from build123d import *

# Parameters (mm, degrees)
ESBO_O1_R                = 6.85
RESSALTO_EXTRUS_O1_DEPTH = 3.2
ESBO_O3_R                = 5.8
RESSALTO_EXTRUS_O2_DEPTH = 15
ESBO_O3_2_R              = 5.8
RESSALTO_EXTRUS_O3_DEPTH = 15


with BuildPart() as part:
    # Esbo_o1 → Ressalto-extrus_o1 (new body)
    with BuildSketch(Plane(origin=(0, 0, 0), x_dir=(1, 0, 0), z_dir=(0, 1, 0))):
        with Locations(Location((0, 0, 0), (0, 0, 270))):
            Circle(ESBO_O1_R)
    extrude(amount=RESSALTO_EXTRUS_O1_DEPTH)

    # Esbo_o3 → Ressalto-extrus_o2 (add)
    with BuildSketch(Plane.XZ):
        with Locations(Location((0, 0, 0), (0, 0, 270))):
            Circle(ESBO_O3_R)
    extrude(amount=RESSALTO_EXTRUS_O2_DEPTH)

    # Esbo_o3_2 → Ressalto-extrus_o3 (add)
    with BuildSketch(Plane.XZ):
        with Locations(Location((0, 0, 0), (0, 0, 270))):
            Circle(ESBO_O3_2_R)
    extrude(amount=RESSALTO_EXTRUS_O3_DEPTH)


solid = part.part
For this review, take the finished solid that the model builds, in its own axes (mm). A direction names the side the tool comes from. Give positions to 0.01 mm unless a question says otherwise; leave off trailing zeros. Loops run counter-clockwise (first coordinate to the right, second up) from the corner with the lowest first, then second, coordinate; pieces in that order, holes last.
Item 1: Take a section at A-A, the plane x = 0. State the section outline as (y, z) points.
Item 2: For line 1 along Y through (x, z) = (-5.5, 2.25); line 2 along Z through (x, y) = (1, 1.25); line 3 along X through (y, z) = (-0.5, 4.5), list the stretches that pass through material, from the lowest coordinate up.
Item 3: Tool access review of faces 1 (the flat face through (2, 0, -6)), 2 (the cylindrical face through (2.058, 1.578, 6.534)): name each direction out of +Z, -Z, +X, -X, +Y, -Y from which nothing blocks a thin tool from reaching the whole face with its end or side.
Item 4: Insertion check: pin 1 (4 mm diameter, centred on y = -0.5, z = 2.5, fed in from -X); pin 2 (3 mm diameter, centred on y = -3.5, z = -1, fed in from -X); pin 3 (1.5 mm diameter, centred on y = -12.5, z = 4, fed in from -X). Each pin has a flat end and moves straight along its axis. Give the tip position at first contact, or say it passes through.
Item 5: Take a section at B-B, the plane z = 0. State the section outline as (x, y) points, and give its area (3 significant figures).
Item 6: Take a section at C-C, the plane y = -13. State the section outline as (x, z) points, and give its area (3 significant figures).
Calculated:
1. outline: (-15, -5.8) - (0, -5.8) - (0, -6.85) - (3.2, -6.85) - (3.2, 6.85) - (0, 6.85) - (0, 5.8) - (-15, 5.8) - close
2. line 1: y = 0 to 3.2
2. line 2: z = -6.78 to 6.78
2. line 3: x = -3.66 to 3.66
3. face 1: -Y
3. face 2: +Y, -Y
4. pin 1: stops at x = -6.83
4. pin 2: stops at x = -5.8
4. pin 3: stops at x = -4.8
5. outline: (-6.85, 0) - (-5.8, 0) - (-5.8, -15) - (5.8, -15) - (5.8, 0) - (6.85, 0) - (6.85, 3.2) - (-6.85, 3.2) - close
5. area: 218 mm2
6. outline: circle Ø11.6 at (0, 0)
6. area: 106 mm2
